Here's how the part is built. I have some questions about the finished solid (model axes, mm). Coordinates: 2 decimals unless noted, no trailing zeros. Write each loop counter-clockwise with the first axis right and the second up, starting at its lowest first coordinate (ties: lowest second). Pieces come first, ordered by that corner, then holes. Notation, with made-up numbers: M 35.25,69 L 59.25,69 A17 ccw 59.25,85 Z; hole C 63.25,7 d2. An arc over 180 degrees is marked long. Use one line per item in the form item = value. Start each with the question number.
1. I want a section at A-A, the plane z = 0. List the corners of the cut face in (x, y) for me, plus the area to 3 significant figures.
2. Please list where these lines run through material, in increasing order: line 1 along Z through (x, y) = (2.5, -0.15); line 2 along X through (y, z) = (0.45, 65); line 3 along X through (y, z) = (-1.05, 73). Write a range as [from, to].
3. I'm going to push flat-ended pins straight in: pin 1 Ø1 at (y, z) = (-0.5, 101) entering from +X; pin 2 Ø3 at (x, z) = (51.27, 51.27) entering from +Y; pin 3 Ø1.2 at (y, z) = (0.5, -68.5) entering from -X; pin 4 Ø1.5 at (x, y) = (-67.5, 1.5) entering from -Z. Where does each tip first touch, or does it pass through?
4. I want a section at C-C, the plane x = 72.5. List the corners of the cut face in (y, z) for me, plus the area to 3 significant figures.
5. I want a section at D-D, the plane z = -102. List the corners of the cut face in (x, y) for me, plus the area to 3 significant figures.
6. I want a section at B-B, the plane y = 0. List the corners of the cut face in (x, z) for me, plus the area to 3 significant figures.
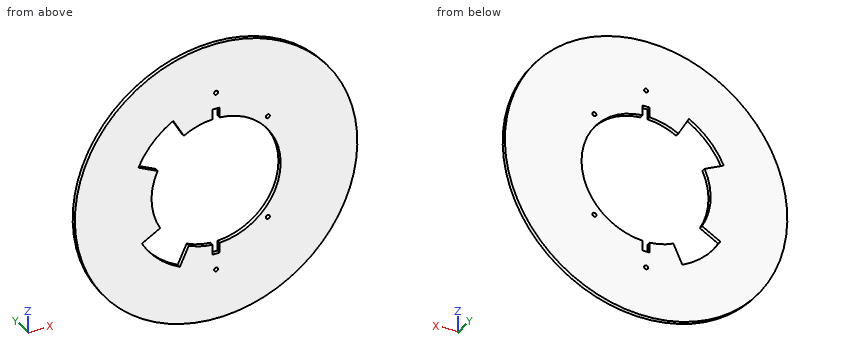
from build123d import *

# Parameters (mm, degrees)
SKETCH1_R           = 140
SKETCH1_R_2         = 64
BOSS_EXTRUDE1_DEPTH = 2
CUT_EXTRUDE1_DEPTH  = 199.030300712
SKETCH4_R           = 2
CUT_EXTRUDE2_DEPTH  = 199.030300712
SKETCH5_R           = 2
CUT_EXTRUDE3_DEPTH  = 199.030300712
SKETCH6_R           = 2
CUT_EXTRUDE4_DEPTH  = 199.030300712
CUT_EXTRUDE6_DEPTH  = 199.030300712


with BuildPart() as part:
    # Sketch1 → Boss-Extrude1 (new, symmetric)
    with BuildSketch(Plane(origin=(0, 0, 0), x_dir=(1, 0, 0), z_dir=(0, 1, 0))):
        with Locations(Location((0, 0, 0), (0, 0, 270))):
            Circle(SKETCH1_R)
        with Locations(Location((0, 0, 0), (0, 0, 270))):
            Circle(SKETCH1_R_2, mode=Mode.SUBTRACT)
    extrude(amount=BOSS_EXTRUDE1_DEPTH, both=True)

    # Sketch2 → Cut-Extrude1 (cut, through all)
    with BuildSketch(Plane(origin=(0, 2, 0), x_dir=(1, 0, 0), z_dir=(0, 1, 0))):
        with BuildLine():
            Line((-3.5, 73.904225212), (0, 73.904225212))
            Line((0, 73.904225212), (3.5, 73.904225212))
            Line((3.5, 73.904225212), (3.5, 63.904225212))
            ThreePointArc((3.5, 63.904225212), (0, 64), (-3.5, 63.904225212))
            Line((-3.5, 63.904225212), (-3.5, 73.904225212))
        make_face()
        with BuildLine():
            Line((3.5, -73.904225212), (3.5, -63.904225212))
            ThreePointArc((3.5, -63.904225212), (0, -64), (-3.5, -63.904225212))
            Line((-3.5, -63.904225212), (-3.5, -73.904225212))
            Line((-3.5, -73.904225212), (0, -73.904225212))
            Line((0, -73.904225212), (3.5, -73.904225212))
        make_face()
    extrude(amount=-CUT_EXTRUDE1_DEPTH, mode=Mode.SUBTRACT)

    # Sketch4 → Cut-Extrude2 (cut, through all)
    with BuildSketch(Plane(origin=(0, 2, 0), x_dir=(1, 0, 0), z_dir=(0, 1, 0))):
        with Locations(Location((-51.265241636, 51.265241636, 0), (0, 0, 270))):
            Circle(SKETCH4_R)
        with Locations(Location((51.265241636, -51.265241636, 0), (0, 0, 90))):
            Circle(SKETCH4_R)
    extrude(amount=-CUT_EXTRUDE2_DEPTH, mode=Mode.SUBTRACT)

    # Sketch5 → Cut-Extrude3 (cut, through all)
    with BuildSketch(Plane(origin=(0, 2, 0), x_dir=(1, 0, 0), z_dir=(0, 1, 0))):
        with Locations(Location((0, -90, 0), (0, 0, 270))):
            Circle(SKETCH5_R)
        with Locations(Location((0, 90, 0), (0, 0, 90))):
            Circle(SKETCH5_R)
    extrude(amount=-CUT_EXTRUDE3_DEPTH, mode=Mode.SUBTRACT)

    # Sketch6 → Cut-Extrude4 (cut, through all)
    with BuildSketch(Plane(origin=(0, 2, 0), x_dir=(1, 0, 0), z_dir=(0, 1, 0))):
        with Locations(Location((-51.265241636, -51.265241636, 0), (0, 0, 270))):
            Circle(SKETCH6_R)
        with Locations(Location((51.265241636, 51.265241636, 0), (0, 0, 90))):
            Circle(SKETCH6_R)
    extrude(amount=-CUT_EXTRUDE4_DEPTH, mode=Mode.SUBTRACT)

    # Sketch7 → Cut-Extrude6 (cut, through all)
    with BuildSketch(Plane(origin=(0, 2, 0), x_dir=(1, 0, 0), z_dir=(0, 1, 0))):
        with BuildLine():
            Line((-27.047568751, 58.00369837), (-35.922552248, 77.036161898))
            ThreePointArc((-35.922552248, 77.036161898), (-57.425167647, 62.668573629), (-73.612159322, 42.5))
            Line((-73.612159322, 42.5), (-55.425625842, 32))
            ThreePointArc((-55.425625842, 32), (-43.237773287, 47.185749556), (-27.047568751, 58.00369837))
        make_face()
        with BuildLine():
            Line((-58.00369837, -27.047568751), (-77.036161898, -35.922552248))
            ThreePointArc((-77.036161898, -35.922552248), (-62.668573629, -57.425167647), (-42.5, -73.612159322))
            Line((-42.5, -73.612159322), (-32, -55.425625842))
            ThreePointArc((-32, -55.425625842), (-47.185749556, -43.237773287), (-58.00369837, -27.047568751))
        make_face()
    extrude(amount=-CUT_EXTRUDE6_DEPTH, mode=Mode.SUBTRACT)


solid = part.part
Answer list:
q1.outline = M -140,-2 L -64,-2 L -64,2 L -140,2 Z; M 64,-2 L 140,-2 L 140,2 L 64,2 Z
q1.area = 608 mm²
q2.line_1 = [-139.98, -73.9], [73.9, 139.98]
q2.line_2 = [-124, -54.77], [-37.53, -3.5], [3.5, 124]
q2.line_3 = [-119.46, -43.54], [-42.15, -3.5], [3.5, 119.46]
q3.pin_1 = 97.47
q3.pin_2 = through
q3.pin_3 = -122.43
q3.pin_4 = -123.06
q4.outline = M -2,-119.77 L 2,-119.77 L 2,119.77 L -2,119.77 Z
q4.area = 958 mm²
q5.outline = M -95.9,-2 L 95.9,-2 L 95.9,2 L -95.9,2 Z
q5.area = 767 mm²
q6.outline = C 0,0 d280; hole M -77.04,35.92 L -58,27.05 A64 ccw -55.43,-32 L -73.61,-42.5 A85 ccw -35.92,-77.04 L -27.05,-58 A64 ccw -3.5,-63.9 L -3.5,-73.9 L 3.5,-73.9 L 3.5,-63.9 A64 ccw 3.5,63.9 L 3.5,73.9 L -3.5,73.9 L -3.5,63.9 A64 ccw -32,55.43 L -42.5,73.61 A85 ccw Z; hole C 0,-90 d4; hole C 0,90 d4; hole C 51.27,-51.27 d4; hole C 51.27,51.27 d4
q6.area = 46,600 mm²
